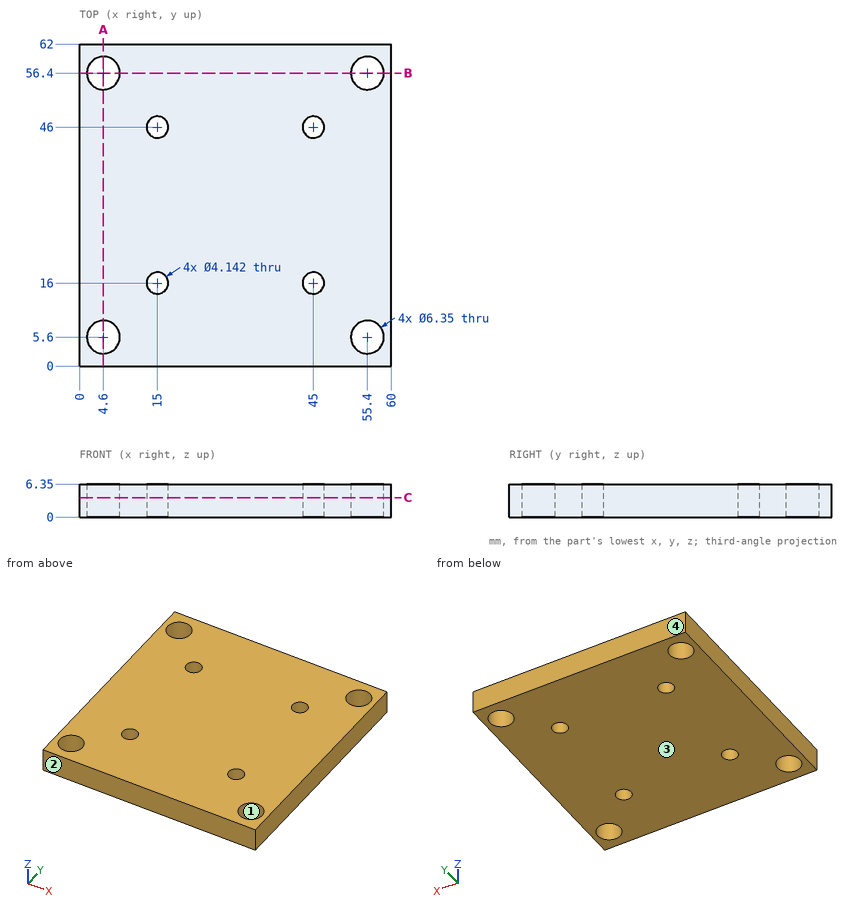
Can you work these out from the drawing? Everything is in mm from the part's minimum corner. Coordinates: 2 decimals unless noted, no trailing zeros. Write each loop counter-clockwise with the first axis right and the second up, starting at its lowest first coordinate (ties: lowest second). Pieces come first, ordered by that corner, then holes. Notation, with made-up numbers: (-7.75, 52.25) - (46.25, 52.25) arc R33 ccw to (46.25, 80.25) - close; hole circle Ø11 at (-5, -25.5). An arc over 180 degrees is marked (long way). Use a Markdown table: item, result.
Q1. Imagine slicing it at B-B (y = 56.4). List the corners of the cut face in (x, z) for me (3 decimals).
Geometry check:
| item | result |
|---|---|
| outline | (0, 0) - (1.425, 0) - (1.425, 6.35) - (0, 6.35) - close; (7.775, 0) - (52.225, 0) - (52.225, 6.35) - (7.775, 6.35) - close; (58.575, 0) - (60, 0) - (60, 6.35) - (58.575, 6.35) - close |
Q2. Imagine slicing it at A-A (x = 4.6). List the corners of the cut face in (y, z) for me (3 decimals), and give its area (3 significant figures).
Geometry check:
| item | result |
|---|---|
| outline | (0, 0) - (2.425, 0) - (2.425, 6.35) - (0, 6.35) - close; (8.775, 0) - (53.225, 0) - (53.225, 6.35) - (8.775, 6.35) - close; (59.575, 0) - (62, 0) - (62, 6.35) - (59.575, 6.35) - close |
| area | 313 mm2 |
Q3. Please list where these lines run through material, in increasing order: L1, parallel to Y at x = 4.6, z = 2.25 (3 decimals); L2, parallel to Y at x = 45, z = 3.25; L3, parallel to X at y = 56, z = 4.
Geometry check:
| item | result |
|---|---|
| L1 | y = 0 to 2.425, 8.775 to 53.225, 59.575 to 62 |
| L2 | y = 0 to 13.93, 18.07 to 43.93, 48.07 to 62 |
| L3 | x = 0 to 1.45, 7.75 to 52.25, 58.55 to 60 |
Q4. Thinking about a two-plate mould opening in Y: for the marked faces 1, 2, 3 and 4, which applies, +Y half, -Y half, draft (parallel to the pull), parting line (faces both ways), or undercut?
Geometry check:
| item | result |
|---|---|
| face 1 | undercut |
| face 2 | -Y half |
| face 3 | draft |
| face 4 | +Y half |
Q5. Imagine slicing it at C-C (z = 3.75). Count the separate pieces of the cut face and the enclosed holes in it, and give its area (3 significant figures).
Geometry check:
| item | result |
|---|---|
| separate pieces | 1 |
| enclosed holes | 8 |
| area | 3,540 mm2 |
